from build123d import *

# Parameters (mm, degrees)
SKETCH_1_R               = 30
EXTRUDE_1_DEPTH          = 2
SKETCH_2_W               = 6
SKETCH_2_H               = 6
EXTRUDE_2_DEPTH          = 2
CUT_EXTRUDE_1_DEPTH      = 43.473521163
CUT_EXTRUDE_1_DEPTH_BACK = 43.473521163
SKETCH_1_10_R            = 1.5
CUT_EXTRUDE_START        = 2
SKETCH_1_11_R            = 2
CUT_EXTRUDE_2_DEPTH      = 2


with BuildPart() as part:
    # 草图1 → 凸台-拉伸1 (new body)
    with BuildSketch(Plane(origin=(0, 0, 0), x_dir=(1, 0, 0), z_dir=(0, 1, 0))):
        with Locations(Location((0, 0, 0), (0, 0, 270))):
            Circle(SKETCH_1_R)
    extrude(amount=EXTRUDE_1_DEPTH)

    # 草图2 → 凸台-拉伸2 (add)
    with BuildSketch(Plane.XZ):
        Rectangle(SKETCH_2_W, SKETCH_2_H)
    extrude(amount=EXTRUDE_2_DEPTH)

    # 草图1<10> → 切除-拉伸1 (cut, two sides: drawn at the far end of the back side and taken through both)
    with BuildSketch(Plane(origin=(0, 0, 0), x_dir=(1, 0, 0), z_dir=(0, 1, 0)).offset(-CUT_EXTRUDE_1_DEPTH_BACK)):
        with Locations(Location((0, 0, 0), (0, 0, 270))):
            Circle(SKETCH_1_10_R)
    extrude(amount=CUT_EXTRUDE_1_DEPTH + CUT_EXTRUDE_1_DEPTH_BACK, mode=Mode.SUBTRACT)

    # 草图1<11> → 切除-拉伸2 (cut)
    with BuildSketch(Plane(origin=(0, 0, 0), x_dir=(1, 0, 0), z_dir=(0, 1, 0)).offset(CUT_EXTRUDE_START)):
        with Locations(Location((0, 0, 0), (0, 0, 270))):
            Circle(SKETCH_1_11_R)
    extrude(amount=-CUT_EXTRUDE_2_DEPTH, mode=Mode.SUBTRACT)


solid = part.part
Model file for the job. Use its own axes, mm. A direction names the side the tool comes from. Round coordinates to 2 decimals unless told otherwise and drop trailing zeros. Order: outer loops, then holes, each group sorted by start corner. A loop starts at its lowest first (then second) coordinate and runs counter-clockwise, first axis right, second up.
(1) Pull direction X, two halves, no side cores. Call faces 5 (the face through (0.45, -1.01, 1.43)), 6 (the face through (0, 2, 6)), 7 (the face through (-3, -1, 0)): released by +X, released by -X, zero draft, split by the parting line, or undercut.
(2) Drill centre lines: line 1 (Z direction, x = 0, y = -0.85); line 2 (X direction, y = 0.7, z = 0). Where is each one in solid material? Low to high.
(3) Band-saw the part on D-D (x = -24). List the corners of the cut face in (y, z).
(4) 3-axis set-ups, long thin cutter, end or side, ignore diameter. For faces 1 (the face through (-2, 1, 0)), 2 (the face through (0, -1, 3)), 3 (the face through (0, -1, -3)), 4 (the face through (3, -1, 0)): which of +Z, -Z, +X, -X, +Y, -Y reach the whole face in a straight line?
(5) Band-saw the part on C-C (x = 0). List the corners of the cut face in (y, z), then the cut area to 3 significant figures.
(6) Band-saw the part on A-A (y = -0.7). List the corners of the cut face in (x, z), then the cut area to 3 significant figures.
(7) Pin check, flat tips, straight feed: pin 1 (1.6 mm diameter, centred on y = -1.5, z = -1, fed in from -X); pin 2 (1.2 mm diameter, centred on x = -1, z = 0, fed in from +Y); pin 3 (1.6 mm diameter, centred on x = 0, y = -1, fed in from +Z); pin 4 (5 mm diameter, centred on x = 0, z = 0, fed in from -Y). Stop position of each tip, or through.
(8) Band-saw the part on B-B (z = 0). List the corners of the cut face in (x, y), then the cut area to 3 significant figures.
Verdict:
1. face 5: undercut
1. face 6: zero draft
1. face 7: released by -X
2. line 1: z = -3 to -1.5, 1.5 to 3
2. line 2: x = -30 to -2, 2 to 30
3. outline: (0, -18) - (2, -18) - (2, 18) - (0, 18) - close
4. face 1: +Y
4. face 2: +Z, +X, -X, -Y
4. face 3: -Z, +X, -X, -Y
4. face 4: +Z, -Z, +X, -Y
5. outline: (-2, -3) - (0, -3) - (0, -30) - (2, -30) - (2, -2) - (0, -2) - (0, -1.5) - (-2, -1.5) - close; (-2, 1.5) - (0, 1.5) - (0, 2) - (2, 2) - (2, 30) - (0, 30) - (0, 3) - (-2, 3) - close
5. area: 118 mm2
6. outline: (-3, -3) - (3, -3) - (3, 3) - (-3, 3) - close; hole circle Ø3 at (0, 0)
6. area: 28.9 mm2
7. pin 1: stops at x = -3
7. pin 2: stops at y = 0
7. pin 3: stops at z = 3
7. pin 4: stops at y = -2
8. outline: (-30, 0) - (-3, 0) - (-3, -2) - (-1.5, -2) - (-1.5, 0) - (-2, 0) - (-2, 2) - (-30, 2) - close; (1.5, -2) - (3, -2) - (3, 0) - (30, 0) - (30, 2) - (2, 2) - (2, 0) - (1.5, 0) - close
8. area: 118 mm2
